from build123d import *

# Parameters (mm, degrees)
BOSS_EXTRUDE1_DEPTH      = 3.175
BOSS_EXTRUDE1_DEPTH_BACK = 0.254
FILLET1_R                = 12.7
SKETCH3_W                = 50.8
SKETCH3_H                = 1.5875
BOSS_EXTRUDE2_DEPTH      = 3.429
CUT_EXTRUDE1_DEPTH       = 305.703453695
CUT_EXTRUDE2_DEPTH       = 305.703453695
CUT_EXTRUDE4_DEPTH       = 305.048068156
BOSS_EXTRUDE3_DEPTH      = 3.175
FILLET2_R                = 12.7
CUT_EXTRUDE5_REACH       = 237.529
SKETCH10_W               = 3.175
SKETCH10_H               = 9.525
SKETCH12_W               = 23.622
SKETCH12_H               = 3.175
BOSS_EXTRUDE4_DEPTH      = 2.54
SKETCH15_W               = 463.920025393
SKETCH15_H               = 26.613528777
CUT_EXTRUDE8_DEPTH       = 237.949226834
BOSS_EXTRUDE5_DEPTH      = 3.429
SKETCH17_W               = 23.622
SKETCH17_H               = 2.54
BOSS_EXTRUDE6_DEPTH      = 3.429
SKETCH18_W               = 3.175
SKETCH18_H               = 3.429
CUT_EXTRUDE9_DEPTH       = 9.525
CUT_EXTRUDE10_DEPTH      = 258.887018005
FILLET3_R                = 12.7
CUT_EXTRUDE11_DEPTH      = 258.887018005


with BuildPart() as part:
    # Sketch1 → Boss-Extrude1 (new, two sides: drawn at the far end of the back side and taken through both)
    with BuildSketch(Plane.XY.offset(-BOSS_EXTRUDE1_DEPTH_BACK)):
        Polygon((-196.85, 0), (-63.5, 230.968975189), (63.5, 230.968975189), (196.85, 0), (167.520606325, 0), (48.835303163, 205.568975189), (-48.835303163, 205.568975189), (-167.520606325, 0), align=None)
    extrude(amount=BOSS_EXTRUDE1_DEPTH + BOSS_EXTRUDE1_DEPTH_BACK)

    # Fillet1
    fillet1_edges = [part.edges().sort_by_distance(p)[0] for p in [
        (167.520606325, 0, 1.4605),
        (48.835303163, 205.568975189, 1.4605),
        (-48.835303163, 205.568975189, 1.4605),
        (-167.520606325, 0, 1.4605),
    ]]
    fillet(fillet1_edges, radius=FILLET1_R)

    # Sketch3 → Boss-Extrude2 (add)
    with BuildSketch(Plane(origin=(0, 0, -0.254), x_dir=(-1, 0, 0), z_dir=(0, 0, -1))):
        Polygon((81.638815329, 202.726625451), (80.264, 201.932875451), (105.664, 157.938784939), (107.038815329, 158.732534939), align=None)
        Polygon((143.614815329, 95.381044601), (142.24, 94.587294601), (167.64, 50.593204089), (169.014815329, 51.386954089), align=None)
        with Locations((0, 231.762725189)):
            Rectangle(SKETCH3_W, SKETCH3_H)
    boss_extrude2 = extrude(amount=-BOSS_EXTRUDE2_DEPTH)

    # Sketch5 → Cut-Extrude1 (cut, through all)
    with BuildSketch(Plane(origin=(0, 0, -0.254), x_dir=(-1, 0, 0), z_dir=(0, 0, -1))):
        Polygon((-175.966912895, 19.672783942), (-185.491912895, 19.672783942), (-187.325, 16.497783942), (-186.309, 16.497783942), (-175.966912895, 16.497783942), align=None)
        Polygon((-186.309, 16.497783942), (-187.325, 16.497783942), (-196.85, 0), (-195.834, 0), align=None)
        Polygon((-121.132358029, 112.096802923), (-129.38125, 116.859302923), (-130.96875, 114.109672266), (-122.719858029, 109.347172266), align=None)
    cut_extrude1 = extrude(amount=-CUT_EXTRUDE1_DEPTH, mode=Mode.SUBTRACT)

    # Sketch4 → Cut-Extrude2 (cut, through all)
    with BuildSketch(Plane(origin=(0, 0, -0.254), x_dir=(-1, 0, 0), z_dir=(0, 0, -1))):
        Polygon((-61.666912895, 230.968975189), (-56.904412895, 222.720083218), (-59.654043552, 221.132583218), (-64.416543552, 229.381475189), (-63.5, 230.968975189), align=None)
    cut_extrude2 = extrude(amount=-CUT_EXTRUDE2_DEPTH, mode=Mode.SUBTRACT)

    # Mirror1: Boss-Extrude2, Cut-Extrude1, Cut-Extrude2 across plane
    add(boss_extrude2.mirror(Plane(origin=(0, 0, 0), x_dir=(0, 0, 1), z_dir=(1, 0, 0))))
    add(cut_extrude1.mirror(Plane(origin=(0, 0, 0), x_dir=(0, 0, 1), z_dir=(1, 0, 0))), mode=Mode.SUBTRACT)
    add(cut_extrude2.mirror(Plane(origin=(0, 0, 0), x_dir=(0, 0, 1), z_dir=(1, 0, 0))), mode=Mode.SUBTRACT)

    # Sketch6 → Cut-Extrude4 (cut, through all)
    with BuildSketch(Plane(origin=(0, 0, -0.254), x_dir=(-1, 0, 0), z_dir=(0, 0, -1))):
        Polygon((-121.326811287, 130.81), (-91.997417612, 130.81), (-52.501477372, 199.218975189), (-41.502954744, 205.568975189), (41.502954744, 205.568975189), (47.852954744, 203.867497817), (52.501477372, 199.218975189), (91.997417612, 130.81), (121.326811287, 130.81), (105.664, 157.938784939), (107.038815329, 158.732534939), (81.638815329, 202.726625451), (80.264, 201.932875451), (64.416543552, 229.381475189), (59.654043552, 221.132583218), (56.904412895, 222.720083218), (61.666912895, 230.968975189), (25.4, 230.968975189), (25.4, 232.556475189), (-25.4, 232.556475189), (-25.4, 230.968975189), (-61.666912895, 230.968975189), (-56.904412895, 222.720083218), (-59.654043552, 221.132583218), (-64.416543552, 229.381475189), (-80.264, 201.932875451), (-81.638815329, 202.726625451), (-107.038815329, 158.732534939), (-105.664, 157.938784939), align=None)
    extrude(amount=-CUT_EXTRUDE4_DEPTH, mode=Mode.SUBTRACT)


with BuildPart() as cut_extrude4_piece_1:
    # of the separate pieces the step leaves, piece 1, a body of its own (cut_extrude4_pieces)
    add(part.part.solids().sort_by_distance((-174.852954744, 0, -0.254))[0])



with BuildPart() as cut_extrude4_piece_2:
    # of the separate pieces the step leaves, piece 2, a body of its own (cut_extrude4_pieces)
    add(part.part.solids().sort_by_distance((195.834, 0, -0.254))[0])


with BuildPart() as cut_extrude4_piece_1_1:
    add(cut_extrude4_piece_1.part)

    add(cut_extrude4_piece_2.part)  # Boss-Extrude3 merges Cut-Extrude4 piece 2
    # Sketch9 → Boss-Extrude3 (add)
    with BuildSketch(Plane(origin=(0, 0, -0.254), x_dir=(-1, 0, 0), z_dir=(0, 0, -1))):
        Polygon((-91.997417612, 130.81), (-106.66211445, 105.41), (106.66211445, 105.41), (91.997417612, 130.81), align=None)
    extrude(amount=-BOSS_EXTRUDE3_DEPTH)

    # Fillet2
    fillet2_edges = [cut_extrude4_piece_1_1.edges().sort_by_distance(p)[0] for p in [
        (-106.66211445, 105.41, 1.3335),
        (106.66211445, 105.41, 1.3335),
    ]]
    fillet(fillet2_edges, radius=FILLET2_R)

    # Sketch10 → Cut-Extrude5 (cut, up to next)
    with BuildSketch(Plane(origin=(0, 0, -0.254), x_dir=(-1, 0, 0), z_dir=(0, 0, -1)), mode=Mode.PRIVATE) as cut_extrude5_sk1:
        with Locations((0, 126.0475)):
            Rectangle(SKETCH10_W, SKETCH10_H)
    cut_extrude5_tool1 = extrude(cut_extrude5_sk1.sketch, amount=-CUT_EXTRUDE5_REACH, mode=Mode.PRIVATE) & cut_extrude4_piece_1_1.part
    add(cut_extrude5_tool1.solids().sort_by_distance((0, 126.0475, -0.254))[0], mode=Mode.SUBTRACT)

    # Sketch12 → Boss-Extrude4 (add)
    with BuildSketch(Plane(origin=(0, 130.81, 0), x_dir=(1, 0, 0), z_dir=(0, 1, 0))):
        with Locations((13.3985, -1.3335)):
            Rectangle(SKETCH12_W, SKETCH12_H)
        with Locations((-13.3985, -1.3335)):
            Rectangle(SKETCH12_W, SKETCH12_H)
    extrude(amount=BOSS_EXTRUDE4_DEPTH)

    # Sketch15 → Cut-Extrude8 (cut, through all)
    with BuildSketch(Plane(origin=(0, 0, -0.254), x_dir=(-1, 0, 0), z_dir=(0, 0, -1))):
        with Locations((4.62960925, 3.191019554)):
            Rectangle(SKETCH15_W, SKETCH15_H)
    extrude(amount=-CUT_EXTRUDE8_DEPTH, mode=Mode.SUBTRACT)

    # Sketch16 → Boss-Extrude5 (add)
    with BuildSketch(Plane(origin=(0, 0, -0.254), x_dir=(-1, 0, 0), z_dir=(0, 0, -1))):
        Polygon((-121.326811287, 130.81), (-94.897086805, 176.587625634), (94.897086805, 176.587625634), (121.326811287, 130.81), (91.997417612, 130.81), (80.232389968, 151.187625634), (-80.232389968, 151.187625634), (-91.997417612, 130.81), align=None)
    extrude(amount=-BOSS_EXTRUDE5_DEPTH)

    # Sketch17 → Boss-Extrude6 (add)
    with BuildSketch(Plane(origin=(0, 0, -0.254), x_dir=(-1, 0, 0), z_dir=(0, 0, -1))):
        with Locations((-13.3985, 177.857625634)):
            Rectangle(SKETCH17_W, SKETCH17_H)
        with Locations((13.3985, 177.857625634)):
            Rectangle(SKETCH17_W, SKETCH17_H)
    extrude(amount=-BOSS_EXTRUDE6_DEPTH)

    # Sketch18 → Cut-Extrude9 (cut)
    with BuildSketch(Plane(origin=(0, 176.587625634, 0), x_dir=(1, 0, 0), z_dir=(0, 1, 0))):
        with Locations((0, -1.4605)):
            Rectangle(SKETCH18_W, SKETCH18_H)
    extrude(amount=-CUT_EXTRUDE9_DEPTH, mode=Mode.SUBTRACT)

    # Sketch19 → Cut-Extrude10 (cut, through all)
    with BuildSketch(Plane(origin=(0, 0, -0.254), x_dir=(-1, 0, 0), z_dir=(0, 0, -1))):
        Polygon((-134.161947492, 57.778891971), (-86.11490379, 140.998812817), (86.11490379, 140.998812817), (134.161947492, 57.778891971), align=None)
    extrude(amount=-CUT_EXTRUDE10_DEPTH, mode=Mode.SUBTRACT)

    # Fillet3
    fillet3_edges = [cut_extrude4_piece_1_1.edges().sort_by_distance(p)[0] for p in [
        (-80.232389968, 151.187625634, 1.4605),
        (80.232389968, 151.187625634, 1.4605),
    ]]
    fillet(fillet3_edges, radius=FILLET3_R)

    # Sketch20 → Cut-Extrude11 (cut, through all)
    with BuildSketch(Plane(origin=(0, 0, -0.254), x_dir=(-1, 0, 0), z_dir=(0, 0, -1))):
        Polygon((93.018969857, 176.587625634), (91.060249362, 173.574435836), (94.601370403, 171.459929994), (96.297026346, 174.162859221), (94.897086805, 176.587625634), align=None)
        Polygon((-94.897086805, 176.587625634), (-96.297026346, 174.162859221), (-94.601370403, 171.459929994), (-91.060249362, 173.574435836), (-93.018969857, 176.587625634), align=None)
    extrude(amount=-CUT_EXTRUDE11_DEPTH, mode=Mode.SUBTRACT)


solid = cut_extrude4_piece_1_1.part
Build history of the part. All positions in model axes, mm. A direction names the side the tool comes from. Coordinates: 2 decimals unless noted, no trailing zeros. Write each loop counter-clockwise with the first axis right and the second up, starting at its lowest first coordinate (ties: lowest second). Pieces come first, ordered by that corner, then holes. Notation, with made-up numbers: (4, 57) -> (17, 57) arc R32 ccw to (17, 90) -> close; hole circle Ø10 at (50.5, 36.5). An arc over 180 degrees is marked (long way). Use CSV: the item, a comma, the result in double quotes. Start each with the question number.
Q1. Drill centre lines: probe 1 along Y at (x, z) = (25, 0.6); probe 2 along Y at (x, z) = (-35.5, 1.6); probe 3 along X at (y, z) = (44, 1.25). Where is each one in solid material? Low to high.
Q2. Flat gauge pins, fed straight in: pin 1 Ø1 at (y, z) = (130, 1.5) entering from -X; pin 2 Ø1 at (y, z) = (97.5, 0) entering from +X; pin 3 Ø1 at (x, z) = (-55, 1) entering from +Y. Where does each tip first touch, or does it go through?
Q3. Pull direction X, two halves, no side cores. Call faces 1 (the flat face through (-15, 152, 3.175)), 2 (the cylindrical face through (79.33, 149.44, 1.48)), 3 (the flat face through (176.44, 35.35, 1.44)): released by +X, released by -X, zero draft, split by the parting line, or undercut.
Q4. Cut at A-A, the plane y = 37. List the corners of the cut face in (x, z) (3 decimals).
Q5. Cut at C-C, the plane y = 88. List the corners of the cut face in (x, z) (3 decimals), then the cut area to 3 significant figures.
Q6. Cut at D-D, the plane x = -137.5. List the corners of the cut face in (y, z) (3 decimals).
Q7. Cut at B-B, the plane x = -53.5. List the corners of the cut face in (y, z) (3 decimals).
Q8. 3-axis set-ups, long thin cutter, end or side, ignore diameter. For faces 4 (the cylindrical face through (-79.17, 149.53, 1.48)), 5 (the flat face through (-15, 152, -0.254)): which of +Z, -Z, +X, -X, +Y, -Y reach the whole face in a straight line?
Checked values:
1,probe 1,"y = 151.19 to 179.13"
1,probe 2,"y = 151.19 to 176.59"
1,probe 3,"x = -171.45 to -142.12, 142.12 to 171.45"
2,pin 1,"stops at x = -122.08"
2,pin 2,"stops at x = 140.85"
2,pin 3,"stops at y = 176.59"
3,face 1,"zero draft"
3,face 2,"undercut"
3,face 3,"released by +X"
4,outline,"(-175.488, -0.254) -> (-146.159, -0.254) -> (-146.159, 3.175) -> (-175.488, 3.175) -> close; (146.159, -0.254) -> (175.488, -0.254) -> (175.488, 3.175) -> (146.159, 3.175) -> close"
5,outline,"(-147.876, -0.254) -> (-116.714, -0.254) -> (-116.714, 3.175) -> (-147.876, 3.175) -> close; (116.714, -0.254) -> (147.876, -0.254) -> (147.876, 3.175) -> (116.714, 3.175) -> close"
5,area,"214 mm²"
6,outline,"(51.997, -0.254) -> (102.797, -0.254) -> (102.797, 3.175) -> (51.997, 3.175) -> close"
7,outline,"(151.188, -0.254) -> (176.588, -0.254) -> (176.588, 3.175) -> (151.188, 3.175) -> close"
8,face 4,"+Z, -Z, -Y"
8,face 5,"-Z, +X, -X, +Y, -Y"
